Autodesk Inventor part; units mm, degrees
ref_plane "YZ Plane" through (0, 0, 0) normal (1, 0, 0) x (0, 1, 0)
ref_plane "XZ Plane" through (0, 0, 0) normal (0, 1, 0) x (-1, 0, 0)
ref_plane "XY Plane" through (0, 0, 0) normal (0, 0, 1) x (1, 0, 0)
sketch "Skizze1" plane through (0, 0, 0) normal (0, 1, 0) x (-1, 0, 0)
  line L0 (39.5556, 0) -> (-37.1227, 0) construction
  line L1 (0, 37.8779) -> (0, -33.8132) construction
  circle A0 centre (35, 0) radius 30.5
  circle A1 centre (35, 0) radius 29
  line L2 (4.7015, 3.5) -> (0, 3.5)
  line L3 (4.7015, -3.5) -> (0, -3.5)
  line L4 (0, 3.5) -> (0, -3.5)
  line L5 (0, 5.5) -> (-5, 5.5)
  line L6 (-5, 5.5) -> (-5, -5.5)
  line L7 (-5, -5.5) -> (0, -5.5)
  line L8 (0, -5.5) -> (0, 5.5)
  line L9 (4.7015, 3.5) -> (6.212, 3.5)
  line L10 (4.7015, -3.5) -> (6.212, -3.5)
  point P0 (0, 0)
  point P1 (0, 3.5)
  dimension "d0" = 61
  dimension "d1" = 35
  dimension "d2" = 1.5
  dimension "d3" = 7
  dimension "d4" = 5
  dimension "d5" = 11
extrude "Extrusion1" add sketch "Skizze1" along normal mid plane 25 contours L9 A1 L10 A0 | A0 L3 L4 L2 | L4 L8 L7 L6 L5 picked at (5.6457, 2.7231)
properties part number "duct_stift"
Verification items for the finished model (mm, model axes). A direction names the side the tool comes from. Round coordinates to 2 decimals unless told otherwise and drop trailing zeros. Order: outer loops, then holes, each group sorted by start corner. A loop starts at its lowest first (then second) coordinate and runs counter-clockwise, first axis right, second up.
1) Material ranges on line 1 (Z direction, x = -4.5, y = 8); line 2 (X direction, y = 6.25, z = 5.25); line 3 (X direction, y = -5, z = 0.25), recorded low to high.
Geometry says:
line 1: z = -3.5 to 3.5
line 2: x = 0 to 5
line 3: x = -6 to 5
2) Tool access check on faces 4 (the flat face through (2, 0, 5.5)), 5 (the flat face through (-3, 0, 3.5)), 6 (the flat face through (-3, 0, -3.5)). Record the directions out of +Z, -Z, +X, -X, +Y, -Y that give a thin tool (end or side, any length) a straight path to the whole face; none if there is none.
Geometry says:
face 4: +Z, +X, -X, +Y, -Y
face 5: +Z, -X, +Y, -Y
face 6: -Z, -X, +Y, -Y
3) Cross-section at B-B, the plane z = -4.5. Record the cut outline in (x, y).
Geometry says:
outline: (0, -12.5) - (5, -12.5) - (5, 12.5) - (0, 12.5) - close
4) Cross-section at C-C, the plane x = -2. Record the cut outline in (y, z), plus the area to 3 significant figures.
Geometry says:
outline: (-12.5, -3.5) - (12.5, -3.5) - (12.5, 3.5) - (-12.5, 3.5) - close
area: 175 mm2
5) Cross-section at A-A, the plane y = -6.75. Record the cut outline in (x, z), plus the area to 3 significant figures.
Geometry says:
outline: (-6.21, -3.5) - (0, -3.5) - (0, -5.5) - (5, -5.5) - (5, 5.5) - (0, 5.5) - (0, 3.5) - (-6.21, 3.5) arc R29 cw to start
area: 97.5 mm2
6) Depth check by flat-ended pin: pin 1 (1.6 mm diameter, centred on y = 5.5, z = -5, fed in from -X); pin 2 (5 mm diameter, centred on x = -1.5, y = 0.5, fed in from -Z); pin 3 (1.5 mm diameter, centred on x = -2, y = 7, fed in from -Z); pin 4 (1.9 mm diameter, centred on x = -3, y = 1, fed in from +Z). Enter the tip coordinate at first touch or a pass-through.
Geometry says:
pin 1: stops at x = 0
pin 2: stops at z = -5.5
pin 3: stops at z = -3.5
pin 4: stops at z = 3.5
7) Draft check along Z on faces 1 (the flat face through (3, 0, -5.5)), 2 (the flat face through (1, -12.5, 0)), 3 (the cylindrical face through (-6, 0, 0)). Enter one of: +Z half, -Z half, draft (parallel to the pull), parting line (faces both ways), or undercut.
Geometry says:
face 1: -Z half
face 2: draft
face 3: undercut
